from build123d import *

# Parameters (mm, degrees)
F1_DEPTH = 1016
F4_DEPTH = 25.4
F2_R     = 3.81
F5_DEPTH = 25.4
F6_DEPTH = 25.4


# Not quite as in the source:
# - a feature names something its author has since deleted; it is built from what else it names


with BuildPart() as f1:
    # F0 (on Top) → F1 (new body)
    with BuildSketch(Plane.XY):
        with BuildLine():
            ThreePointArc((12.7, 6.35), (10.8401280605, 10.8401280605), (6.35, 12.7))
            Line((6.35, 12.7), (-6.35, 12.7))
            ThreePointArc((-6.35, 12.7), (-10.8401280605, 10.8401280605), (-12.7, 6.35))
            Line((-12.7, 6.35), (-12.7, -6.35))
            ThreePointArc((-12.7, -6.35), (-10.8401280605, -10.8401280605), (-6.35, -12.7))
            Line((-6.35, -12.7), (6.35, -12.7))
            ThreePointArc((6.35, -12.7), (10.8401280605, -10.8401280605), (12.7, -6.35))
            Line((12.7, -6.35), (12.7, 6.35))
        make_face()
    extrude(amount=F1_DEPTH)

    # F3 (on face) → F4 (cut)
    with BuildSketch(Plane.YZ.offset(12.7)):
        with BuildLine():
            ThreePointArc((3.81, 1003.3), (2.6940768363, 1005.9940768363), (0, 1007.11))
            ThreePointArc((0, 1007.11), (-2.6940768363, 1000.6059231637), (3.81, 1003.3))
        make_face()
    extrude(amount=-F4_DEPTH, mode=Mode.SUBTRACT)

    # F2 (on face) → F5 (cut)
    with BuildSketch(Plane.XZ.offset(12.7)):
        with BuildLine():
            ThreePointArc((3.81, 1003.3), (2.6940768363, 1005.9940768363), (0, 1007.11))
            ThreePointArc((0, 1007.11), (-2.6940768363, 1000.6059231637), (3.81, 1003.3))
        make_face()
        with Locations((0, 876.3)):
            Circle(F2_R)
        with Locations((0, 647.7)):
            Circle(F2_R)
        with Locations((0, 419.1)):
            Circle(F2_R)
    extrude(amount=-F5_DEPTH, mode=Mode.SUBTRACT)

    # F2 (on face) → F6 (cut)
    with BuildSketch(Plane.XZ.offset(12.7)):
        with Locations((0, 190.5)):
            Circle(F2_R)
    extrude(amount=-F6_DEPTH, mode=Mode.SUBTRACT)


solid = f1.part
Can you work these out from the model? Positions are in its coordinate system, mm. Give positions to 0.01 mm unless a question says otherwise; leave off trailing zeros. Order: outer loops, then holes, each group sorted by start corner. A loop starts at its lowest first (then second) coordinate and runs counter-clockwise, first axis right, second up. Notation, with made-up numbers: M 31.5,-2 L 51.5,-2 A23 cw 51.5,37 Z; hole C 41.5,88 d8. An arc over 180 degrees is marked long. One line per question, with ' | ' between items.
Item 1: I'm going to push flat-ended pins straight in: pin 1 Ø2 at (x, z) = (-9.5, 853.5) entering from -Y; pin 2 Ø1.5 at (y, z) = (8, 268.5) entering from -X; pin 3 Ø6 at (x, z) = (0, 647.7) entering from -Y. Where does each tip first touch, or does it pass through?
Answer block:
pin 1: stops at y = -12.32 | pin 2: stops at x = -12.64 | pin 3: passes through
Item 2: Suppose I cut it at A-A, the plane z = 938. Write out the boundary of the cut face in (x, y), then the cut area to 3 significant figures.
Answer block:
outline: M -12.7,-6.35 A6.35 ccw -6.35,-12.7 L 6.35,-12.7 A6.35 ccw 12.7,-6.35 L 12.7,6.35 A6.35 ccw 6.35,12.7 L -6.35,12.7 A6.35 ccw -12.7,6.35 Z | area: 611 mm2
Item 3: Please list where these lines run through material, in increasing order: L1, parallel to Z at x = 0, y = 5.5; L2, parallel to X at y = -2.25, z = 190.5; L3, parallel to X at y = -7.5, z = 876.3 (3 decimals).
Answer block:
L1: z = 0 to 186.69, 194.31 to 415.29, 422.91 to 643.89, 651.51 to 872.49, 880.11 to 999.49, 1007.11 to 1016 | L2: x = -12.7 to -3.81, 3.81 to 12.7 | L3: x = -12.595 to -3.81, 3.81 to 12.595
